Autodesk Fusion 360 part; units mm, degrees
sketch "Sketch1" plane through (0, 0, 0) normal (0, 0, 1) x (1, 0, 0)
  line L0 (-15, -15) -> (15, -15)
  line L1 (15, -15) -> (15, 15)
  line L2 (15, 15) -> (-15, 15)
  line L3 (-15, 15) -> (-15, -15)
  line L4 (-15, -15) -> (15, 15) construction
  line L5 (15, -15) -> (-15, 15) construction
  line L6 (-25, 25) -> (25, 25)
  line L7 (25, 25) -> (25, -25)
  line L8 (25, -25) -> (-25, -25)
  line L9 (-25, -25) -> (-25, 25)
  line L10 (15, -15) -> (25, -25) construction
  line L11 (-25, 25) -> (-15, 15) construction
  line L12 (15, 15) -> (25, 25) construction
  line L13 (-15, -15) -> (-25, -25) construction
  dimension "d1" = 30
  dimension "d2" = 30
  dimension "d23" = 10
  dimension "d24" = 10
  dimension "d25" = 10
  dimension "d26" = 10
extrude "Extrude1" add sketch "Sketch1" along normal blind 5 contours L0 L1 L2 L3
ref_plane "WorkPlane1" through (0, 0, 0) normal (0.7071, 0.7071, 0) x (-0.7071, 0.7071, 0)
ref_plane "WorkPlane2" through (0, 0, 0) normal (0.7071, -0.7071, 0) x (0.7071, 0.7071, 0)
sketch "Sketch2" plane through (0, 0, 0) normal (0.7071, 0.7071, 0) x (-0.7071, 0.7071, 0)
  circle A0 centre (0, -15) radius 5
  line L0 (2.5, -10.6699) -> (2.5, -2.5)
  line L1 (-2.5, -10.6699) -> (-2.5, -2.5)
  arc A1 (5, 0) -> (2.5, -2.5) centre (5, -2.5) ccw
  arc A2 (-2.5, -2.5) -> (-5, 0) centre (-5, -2.5) ccw
  line L2 (0, 0) -> (0, -15) construction
  line L3 (0, -7.5) -> (2.5, -7.5) construction
  line L4 (0, -7.5) -> (-2.5, -7.5) construction
  line L5 (21.2132, 0) -> (0, 0)
  line L6 (0, 0) -> (-21.2132, 0)
  line L7 (5, -2.5) -> (-5, -2.5) construction
  arc A3 (2.5, -9.4098) -> (3.3333, -11.2732) centre (5, -9.4098) ccw
  arc A4 (-3.3333, -11.2732) -> (-2.5, -9.4098) centre (-5, -9.4098) ccw
  line L8 (-17.2446, 0) -> (-17.2446, -26.2222)
  line L9 (-17.2446, -26.2222) -> (15.3661, -26.2222)
  line L10 (15.3661, -26.2222) -> (15.3661, 0)
  line L11 (0, -20) -> (0, -26.2222)
  dimension "d7" = 10
  dimension "d8" = 5
  dimension "d9" = 15
  dimension "d14" = 2.5
extrude "Extrude2" add sketch "Sketch2" along normal blind 25 and the other way blind 5 contours A0 | A0 L0 A3 | A0 L0 L1 A1 A2 L5 L6 | A0 L1 A4
sketch "Sketch3" plane through (0, 0, 0) normal (0.7071, -0.7071, 0) x (0.7071, 0.7071, 0)
  circle A0 centre (0, -15) radius 5
  line L0 (0, 0) -> (0, -15) construction
  line L1 (-2.5, -2.5) -> (-2.5, -9.4098)
  line L2 (2.5, -2.5) -> (2.5, -9.4098)
  line L3 (-21.2132, 0) -> (0, 0)
  line L4 (0, -5.6591) -> (2.5, -5.6591) construction
  line L5 (0, -5.6591) -> (-2.5, -5.6591) construction
  arc A1 (-3.3333, -11.2732) -> (-2.5, -9.4098) centre (-5, -9.4098) ccw
  arc A2 (2.5, -9.4098) -> (3.3333, -11.2732) centre (5, -9.4098) ccw
  arc A3 (-2.5, -2.5) -> (-5, 0) centre (-5, -2.5) ccw
  line L6 (0, 0) -> (16.2132, 0)
  arc A4 (5, 0) -> (2.5, -2.5) centre (5, -2.5) ccw
  line L7 (-15.7318, 0) -> (-15.7318, -22.3804)
  line L8 (-15.7318, -22.3804) -> (13.46, -22.3804)
  line L9 (13.46, -22.3804) -> (13.46, 0)
  line L10 (0, -20) -> (0, -22.3804)
  line L11 (0, 0) -> (0, -26.2222)
  dimension "d12" = 15
  dimension "d13" = 10
  dimension "d15" = 5
  dimension "d16" = 2.5
extrude "Extrude3" add sketch "Sketch3" along normal blind 25 and the other way blind 5 contours A0 L11 | A0 L2 A2 L6 A4 L11 | A0 L11 | A0 L1 L3 A1 A3 L11
extrude "Extrude4" cut sketch "Sketch1" against normal blind 20
extrude "Extrude5" cut sketch "Sketch2" along normal mid plane 30 contours A0 L0 A1 L5 A3 L9 L10 L11
extrude "Extrude6" cut sketch "Sketch3" along normal mid plane 30 contours A0 L1 L3 A1 A3 L7 L8 L10 L11
equation "d23 = d26"
equation "d24 = d26"
equation "d25 = d26"
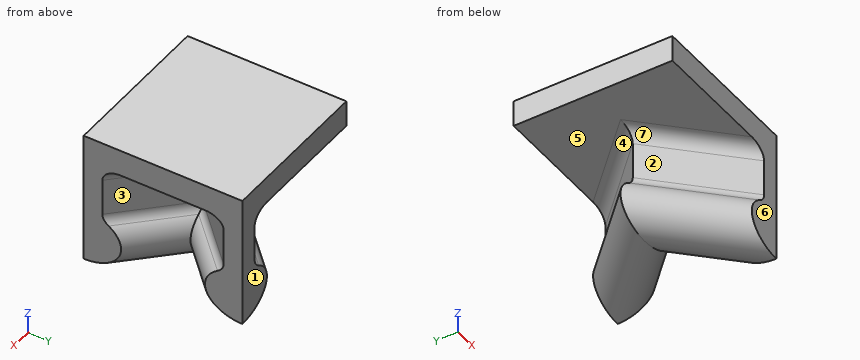
Can you work these out from the model? Positions are in its coordinate system, mm. Face numbers are marked on the shaded views. A direction names the side the tool comes from. Round coordinates to 2 decimals unless told otherwise and drop trailing zeros. Write each loop counter-clockwise with the first axis right and the second up, starting at its lowest first coordinate (ties: lowest second). Pieces come first, ordered by that corner, then holes. Notation, with made-up numbers: (22, 43.25) -> (59, 43.25) arc R22 cw to (59, 59.25) -> close; hole circle Ø1 at (43, -12). An arc over 180 degrees is marked (long way). Use one line per item in the form item = value. Start each with the question number.
Q1. I'm going to push flat-ended pins straight in: P1, Ø2, axis at y = 2.5, z = -10.5, coming from the +X side; P2, Ø1.5, axis at x = -5, z = -6, coming from the +Y side; P3, Ø1.5, axis at y = -7, z = -16.5, coming from the +X side; P4, Ø3, axis at x = -6.5, y = 6.5, coming from the -Z side. Where does each tip first touch, or does it pass through?
Q2. We'd pull the mould along Z, two halves only. Please class the marked faces 5, 6 and 7: +Z half, -Z half, draft (parallel to the pull), parting line (faces both ways), or undercut.
Q3. Which directions (+Z, -Z, +X, -X, +Y, -Y) give clear straight access to the entire face, cutting with the end or side of a thin tool? Please do the marked faces 1, 2, 3 and 4.
Q4. Imagine slicing it at C-C (z = -14.5). Please give me the cut outline in (x, y).
Q5. Imagine slicing it at B-B (x = -10.5). Please give me the cut outline in (y, z).
Q6. Imagine slicing it at A-A (z = -9). Please give me the cut outline in (x, y), then the cut area to 3 significant figures.
Q7. If I drill on probe 1 along Z at (x, y) = (-11, 13.5); probe 2 along Z at (x, y) = (10, -5); probe 3 along Y at (x, z) = (9, -2.75), over which ranges is the centre line in solid material (lowest first)? Write a range as [from, to].
Worked out:
q1.P1 = 7.86
q1.P2 = through
q1.P3 = 14.55
q1.P4 = 0
q2.face_5 = -Z half
q2.face_6 = draft
q2.face_7 = undercut
q3.face_1 = +Z, -Z, +X, -X, +Y
q3.face_2 = -X, -Y
q3.face_3 = +X
q3.face_4 = -X, +Y
q4.outline = (-7.04, 0) -> (7.96, -15) -> (15, -15) -> (15, -7.96) -> (7.04, 0) -> (15, 7.96) -> (15, 15) -> (7.96, 15) -> close
q5.outline = (-15, 0) -> (15, 0) -> (15, 5) -> (-15, 5) -> close
q6.outline = (-3.54, 0) -> (11.46, -15) -> (15, -15) -> (15, -11.46) -> (3.54, 0) -> (15, 11.46) -> (15, 15) -> (11.46, 15) -> close
q6.area = 200 mm^2
q7.probe_1 = [0, 5]
q7.probe_2 = [-18.54, -11.46], [-0.47, 5]
q7.probe_3 = [-12.54, -5.46], [5.46, 12.54]
